Here's how the part is built. I have some questions about the finished solid (model axes, mm). A direction names the side the tool comes from. Coordinates: 2 decimals unless noted, no trailing zeros. Use a Markdown table: item, result.
```python
from build123d import *


with BuildPart() as part:
    # Sketch1 → Revolve1 (revolve)
    with BuildSketch(Plane(origin=(0, 0, 0), x_dir=(0, 0, -1), z_dir=(1, 0, 0)), mode=Mode.PRIVATE) as revolve1_sk:
        with BuildLine():
            Line((-9.525, 6.35), (9.525, 6.35))
            Line((9.525, 6.35), (9.525, 11.1125))
            Line((9.525, 11.1125), (4.7625, 11.1125))
            Line((4.7625, 11.1125), (4.7625, 38.1))
            Line((4.7625, 38.1), (9.525, 38.1))
            Line((9.525, 38.1), (9.525, 50.8))
            Line((9.525, 50.8), (6.35, 50.8))
            ThreePointArc((6.35, 50.8), (0, 44.45), (-6.35, 50.8))
            Line((-6.35, 50.8), (-9.525, 50.8))
            Line((-9.525, 50.8), (-9.525, 38.1))
            Line((-9.525, 38.1), (-4.7625, 38.1))
            Line((-4.7625, 38.1), (-4.7625, 11.1125))
            Line((-4.7625, 11.1125), (-9.525, 11.1125))
            Line((-9.525, 11.1125), (-9.525, 6.35))
        make_face()
    revolve(revolve1_sk.sketch.rotate(Axis((0, 0, 17.864143374), (0, 0, -1)), 90), axis=Axis((0, 0, 17.864143374), (0, 0, -1)))


solid = part.part
```
1. Will these pins go through, and if not, where does the flat tip stop? pin 1 Ø5 at (x, z) = (7, -7.5) entering from -Y; pin 2 Ø8 at (y, z) = (-19.5, -4) entering from -X; pin 3 Ø1.5 at (x, z) = (32, 4) entering from -Y.
Answers follow:
| item | result |
|---|---|
| pin 1 | stops at y = -50.6 |
| pin 2 | stops at x = -48.13 |
| pin 3 | stops at y = -34.06 |
2. We'd pull the mould along X, two halves only. Please class faces 4 (the face through (-5.04, 3.86, -0.13)), 5 (the face through (-8.259, 37.194, 7.11)), 6 (the face through (-7, -38, -9.525)), 7 (the face through (-40.313, 30.911, 7.96)): +X half, -X half, draft (parallel to the pull), parting line (faces both ways), or undercut.
Answers follow:
| item | result |
|---|---|
| face 4 | undercut |
| face 5 | undercut |
| face 6 | draft |
| face 7 | parting line |
3. I need wall thicknesses on probe 1 along Y at (x, z) = (0, 7.5); probe 2 along X at (y, z) = (6.5, -5.75); probe 3 along Z at (x, y) = (19.5, -2.5). Which ranges of each line are inside material? Lowest first, please.
Answers follow:
| item | result |
|---|---|
| probe 1 | y = -50.8 to -38.1, -11.11 to -6.35, 6.35 to 11.11, 38.1 to 50.8 |
| probe 2 | x = -47.66 to -37.54, -9.01 to 9.01, 37.54 to 47.66 |
| probe 3 | z = -4.76 to 4.76 |
4. Which directions (+Z, -Z, +X, -X, +Y, -Y) give clear straight access to the entire face, cutting with the end or side of a thin tool? Please do faces 1 (the face through (-8.2, -7.5, -7.1)), 2 (the face through (-40.313, 30.911, -7.915)), 3 (the face through (8, 8, 4.762)).
Answers follow:
| item | result |
|---|---|
| face 1 | -Z |
| face 2 | +Z, -Z |
| face 3 | +Z |
